Autodesk Inventor part; units mm, degrees
ref_plane "YZ Plane" through (0, 0, 0) normal (1, 0, 0) x (0, 1, 0)
ref_plane "XZ Plane" through (0, 0, 0) normal (0, 1, 0) x (-1, 0, 0)
ref_plane "XY Plane" through (0, 0, 0) normal (0, 0, 1) x (1, 0, 0)
sketch "Sketch1" plane through (0, 0, 0) normal (0, 0, 1) x (1, 0, 0)
  line L0 (27, 12) -> (0, 12)
  line L1 (0, 12) -> (0, 0)
  line L2 (27, 12) -> (27, 9.5)
  line L3 (27, 9.5) -> (23.5, 9.5)
  line L4 (23.5, 2.5) -> (27, 2.5)
  line L5 (27, 2.5) -> (27, 0)
  line L6 (27, 0) -> (23.5, 0)
  line L7 (23.5, 7.25) -> (27, 7.25)
  line L8 (27, 7.25) -> (27, 4.75)
  line L9 (27, 4.75) -> (23.5, 4.75)
  line L10 (23.5, 2.5) -> (23.5, 4.75)
  line L11 (23.5, 7.25) -> (23.5, 9.5)
  line L12 (0, 0) -> (27, 0)
  dimension "d2" = 2.5
  dimension "d4" = 2.5
  dimension "d8" = 2.5
  dimension "d9" = 2.25
  dimension "d10" = 7
  dimension "d11" = 27
  dimension "d12" = 12
  dimension "d13" = 3.5
  dimension "d14" = 3.5
  dimension "d15" = 3.5
extrude "Extrusion1" add sketch "Sketch1" along normal blind 5
equation "\"d4\" = d2"
equation "\"d8\" = d2"
equation "\"d9\" = -0.5 * d8 + 0.5 * d10"
equation "\"d14\" = d13"
properties part number "FVT LITTLEBEE BLHeli 20A ESC" material "Nylon 6/6"
Check sheet for the modelled part. Datum: model origin and axes. Units: mm. A direction names the side the tool comes from. Round coordinates to 2 decimals unless told otherwise and drop trailing zeros. Write each loop counter-clockwise with the first axis right and the second up, starting at its lowest first coordinate (ties: lowest second). Pieces come first, ordered by that corner, then holes. Notation, with made-up numbers: M 12.25,48 L 55.25,48 A23 cw 55.25,77 Z; hole C -19,-24.75 d5. An arc over 180 degrees is marked long. Write item = value, one per line. Start each with the question number.
1. Release check for a two-part mould opening along Y. For faces 3 (the flat face through (25, 7.25, 2)), 4 (the flat face through (27, 6, 2)), 5 (the flat face through (14, 0, 2)) record: pulls with the +Y half, pulls with the -Y half, needs draft (parallel to the pull), parting line crosses it, or undercut.
2. Tool access check on faces 1 (the flat face through (23.5, 8, 2)), 2 (the flat face through (13, 6, 0)). Record the directions out of +Z, -Z, +X, -X, +Y, -Y that give a thin tool (end or side, any length) a straight path to the whole face; none if there is none.
3. Section check A-A, the plane x = 25.75. Record the cut outline in (y, z).
4. Scan lines: line 1 (Y direction, x = 23.75, z = 2); line 2 (X direction, y = 8.5, z = 4.1). Record each from-to range of solid material in increasing order. Write a range as [from, to].
5. Section check C-C, the plane y = 8.75. Record the cut outline in (x, z).
6. Gauge pin test, flat ends, axial feed: pin 1 (1.5 mm diameter, centred on y = 8, z = 0.5, fed in from -X); pin 2 (0.7 mm diameter, centred on y = 8, z = 2, fed in from +X). Record the tip position at first contact, or that the pin passes through.
7. Section check B-B, the plane z = 2.4. Record the cut outline in (x, y), then the cut area to 3 significant figures.
Results found:
q1.face_3 = undercut
q1.face_4 = needs draft
q1.face_5 = pulls with the -Y half
q2.face_1 = +Z, -Z, +X
q2.face_2 = -Z, +X, -X, +Y, -Y
q3.outline = M 0,0 L 2.5,0 L 2.5,5 L 0,5 Z; M 4.75,0 L 7.25,0 L 7.25,5 L 4.75,5 Z; M 9.5,0 L 12,0 L 12,5 L 9.5,5 Z
q4.line_1 = [0, 2.5], [4.75, 7.25], [9.5, 12]
q4.line_2 = [0, 23.5]
q5.outline = M 0,0 L 23.5,0 L 23.5,5 L 0,5 Z
q6.pin_1 = 0
q6.pin_2 = 23.5
q7.outline = M 0,0 L 27,0 L 27,2.5 L 23.5,2.5 L 23.5,4.75 L 27,4.75 L 27,7.25 L 23.5,7.25 L 23.5,9.5 L 27,9.5 L 27,12 L 0,12 Z
q7.area = 308 mm^2
